Part model, mm, in its own coordinate system. A direction names the side the tool comes from. Give positions to 0.01 mm unless a question says otherwise; leave off trailing zeros. Loops run counter-clockwise (first coordinate to the right, second up) from the corner with the lowest first, then second, coordinate; pieces in that order, holes last. Notation, with made-up numbers: (58.25, 16) -> (85.25, 16) arc R24 cw to (85.25, 28) -> close; hole circle Ø11 at (-5.5, 2.25). An arc over 180 degrees is marked (long way). One line per question, with ' | ' between items.
```python
from build123d import *

# Parameters (mm, degrees)
SKETCH_1_W               = 45.9
SKETCH_1_H               = 49.9
EXTRUDE_1_DEPTH          = 6
SKETCH_2_R               = 1.9
EXTRUDE_2_DEPTH          = 8.9
EXTRUDE_START            = -8.9
SKETCH_3_R               = 1.9
EXTRUDE_3_DEPTH          = 8.9
FILLET_3_R               = 10
CUT_EXTRUDE_START        = -10
SKETCH_6_R               = 1.9
CUT_EXTRUDE_2_DEPTH      = 10
SKETCH_7_W               = 45.9
SKETCH_7_H               = 49.9
CUT_EXTRUDE_3_DEPTH      = 5
FILLET_4_R               = 4
SKETCH_8_W               = 28.1
SKETCH_8_H               = 49.9
EXTRUDE_5_DEPTH          = 5
FILLET_5_R               = 2
SKETCH_11_R              = 2.25
CUT_EXTRUDE_4_DEPTH      = 31
CUT_EXTRUDE_1_DEPTH      = 66
CUT_EXTRUDE_1_DEPTH_BACK = 70


with BuildPart() as part:
    # 草图1 → 凸台-拉伸1 (new body)
    with BuildSketch(Plane.XY):
        with Locations((22.95, -24.95)):
            Rectangle(SKETCH_1_W, SKETCH_1_H)
    extrude(amount=EXTRUDE_1_DEPTH)

    # 草图2 → 凸台-拉伸2 (add)
    with BuildSketch(Plane(origin=(45.9, 0, 0), x_dir=(0, 0, -1), z_dir=(1, 0, 0))):
        with BuildLine():
            Line((-6, 0), (-17.3, 0))
            ThreePointArc((-17.3, 0), (-20.410567122, 4.633542967), (-24.02783532, 8.883333436))
            ThreePointArc((-24.02783532, 8.883333436), (-33.92465453, 9.113485719), (-34.154806758, -0.783333492))
            ThreePointArc((-34.154806758, -0.783333492), (-24.472236128, -24.949999926), (-34.154806656, -49.116666401))
            ThreePointArc((-34.154806656, -49.116666401), (-33.924654493, -59.013485754), (-24.027835147, -58.783333255))
            ThreePointArc((-24.027835147, -58.783333255), (-20.410567046, -54.533542867), (-17.3, -49.9))
            Line((-17.3, -49.9), (-6, -49.9))
            Line((-6, -49.9), (-6, 0))
        make_face()
        with Locations(Location((-16.972236128, -24.95, 0), (0, 0, 90))):
            Circle(SKETCH_2_R, mode=Mode.SUBTRACT)
        with Locations(Location((-29.420197927, 5.1020382, 0), (0, 0, 90))):
            Circle(SKETCH_2_R, mode=Mode.SUBTRACT)
        with Locations(Location((-29.420197927, -55.0020382, 0), (0, 0, 90))):
            Circle(SKETCH_2_R, mode=Mode.SUBTRACT)
    extrude(amount=-EXTRUDE_2_DEPTH)

    # 草图3 → 凸台-拉伸3 (add)
    with BuildSketch(Plane.ZY.offset(EXTRUDE_START)):
        with BuildLine():
            Line((6, -49.9), (17.3, -49.9))
            ThreePointArc((17.3, -49.9), (62.08503163, -73.880290206), (104.061658089, -45.267072848))
            ThreePointArc((104.061658089, -45.267072848), (100.098824974, -34.670094153), (89.501846395, -38.63292758))
            ThreePointArc((89.501846395, -38.63292758), (26.472236128, -24.950000045), (89.501846358, -11.267072337))
            ThreePointArc((89.501846358, -11.267072337), (100.09882522, -15.229905735), (104.061657827, -4.632926576))
            ThreePointArc((104.061657827, -4.632926576), (62.085031314, 23.980290223), (17.3, 0))
            Line((17.3, 0), (6, 0))
            Line((6, 0), (6, -49.9))
        make_face()
        with Locations(Location((90.93848789, 6.516251763, 0), (0, 0, 270))):
            Circle(SKETCH_3_R, mode=Mode.SUBTRACT)
        with Locations(Location((28.005984365, -56.416251763, 0), (0, 0, 270))):
            Circle(SKETCH_3_R, mode=Mode.SUBTRACT)
        with Locations(Location((16.972236128, -24.95, 0), (0, 0, 90))):
            Circle(SKETCH_3_R, mode=Mode.SUBTRACT)
        with Locations(Location((59.472236128, -69.45, 0), (0, 0, 270))):
            Circle(SKETCH_3_R, mode=Mode.SUBTRACT)
        with Locations(Location((90.93848789, -56.416251763, 0), (0, 0, 270))):
            Circle(SKETCH_3_R, mode=Mode.SUBTRACT)
        with Locations(Location((28.005984365, 6.516251763, 0), (0, 0, 270))):
            Circle(SKETCH_3_R, mode=Mode.SUBTRACT)
        with Locations(Location((59.472236128, 19.55, 0), (0, 0, 270))):
            Circle(SKETCH_3_R, mode=Mode.SUBTRACT)
    extrude(amount=EXTRUDE_3_DEPTH)

    # 圆角3
    fillet_3_edges = [part.edges().sort_by_distance(p)[0] for p in [
        (41.45, 0, 17.3),
        (41.45, -49.9, 17.3),
        (4.45, -49.9, 17.3),
        (4.45, 0, 17.3),
    ]]
    fillet(fillet_3_edges, radius=FILLET_3_R)

    # 草图6 → 切除-拉伸2 (cut)
    # profile 1 of 2: a face of its own
    with BuildSketch(Plane.ZY.offset(CUT_EXTRUDE_START)):
        with BuildLine():
            ThreePointArc((104.061657942, -4.632926829), (85.981321722, 16.260051941), (59.472232168, 24.05))
            ThreePointArc((59.472232168, 24.05), (65.12908684, 21.706854481), (67.472232822, 16.05))
            ThreePointArc((67.472232822, 16.05), (65.129087169, 10.393145848), (59.472233099, 8.05))
            ThreePointArc((59.472233099, 8.05), (77.32529362, 2.803708548), (89.501846738, -11.267073171))
            ThreePointArc((89.501846738, -11.267073171), (100.098825511, -15.229905602), (104.061657942, -4.632926829))
        make_face()
        with Locations((90.93848789, 6.516251763)):
            Circle(SKETCH_6_R, mode=Mode.SUBTRACT)
    # profile 2 of 2: a face of its own
    with BuildSketch(Plane.ZY.offset(CUT_EXTRUDE_START)):
        with BuildLine():
            ThreePointArc((89.501846738, -38.632926829), (77.325293679, -52.70370851), (59.472233238, -57.95))
            ThreePointArc((59.472233238, -57.95), (65.129087219, -60.293145898), (67.472232822, -65.95))
            ThreePointArc((67.472232822, -65.95), (65.129086835, -71.606854486), (59.472232153, -73.95))
            ThreePointArc((59.472232153, -73.95), (85.981321716, -66.160051945), (104.061657942, -45.267073171))
            ThreePointArc((104.061657942, -45.267073171), (100.098825511, -34.670094398), (89.501846738, -38.632926829))
        make_face()
        with Locations((90.93848789, -56.416251763)):
            Circle(SKETCH_6_R, mode=Mode.SUBTRACT)
    extrude(amount=CUT_EXTRUDE_2_DEPTH, mode=Mode.SUBTRACT)


with BuildPart() as cut_extrude_2_kept_piece:
    # of the separate pieces the step leaves, the one the design keeps (cut_extrude_2_pieces_kept)
    add(part.part.solids().sort_by_distance((0, 0, 11.938064209))[0])

    # 草图7 → 切除-拉伸3 (cut)
    with BuildSketch(Plane(origin=(0, 0, 0), x_dir=(-1, 0, 0), z_dir=(0, 0, -1))):
        with Locations((-22.95, -24.95)):
            Rectangle(SKETCH_7_W, SKETCH_7_H)
    extrude(amount=-CUT_EXTRUDE_3_DEPTH, mode=Mode.SUBTRACT)

    # 圆角4
    fillet_4_edges = [cut_extrude_2_kept_piece.edges().sort_by_distance(p)[0] for p in [
        (45.9, -24.95, 5),
        (0, -24.95, 5),
    ]]
    fillet(fillet_4_edges, radius=FILLET_4_R)

    # 草图8 → 凸台-拉伸5 (add)
    with BuildSketch(Plane.XY.offset(6)):
        with Locations((22.95, -24.95)):
            Rectangle(SKETCH_8_W, SKETCH_8_H)
    extrude(amount=EXTRUDE_5_DEPTH)

    # 圆角5
    fillet_5_edges = [cut_extrude_2_kept_piece.edges().sort_by_distance(p)[0] for p in [
        (37, -24.95, 11),
        (8.9, -24.95, 11),
    ]]
    fillet(fillet_5_edges, radius=FILLET_5_R)

    # 草图11 → 切除-拉伸4 (cut)
    with BuildSketch(Plane.XY.offset(11)):
        with Locations((22.95, -7.7)):
            Circle(SKETCH_11_R)
        with Locations((22.95, -42.2)):
            Circle(SKETCH_11_R)
    extrude(amount=-CUT_EXTRUDE_4_DEPTH, mode=Mode.SUBTRACT)

    # 草图4 → 切除-拉伸1 (cut, two sides: drawn at the far end of the back side and taken through both)
    with BuildSketch(Plane.XY.offset(6).offset(-CUT_EXTRUDE_1_DEPTH_BACK)):
        with BuildLine():
            ThreePointArc((28.95, -24.95), (27.192640687, -20.707359313), (22.95, -18.95))
            Line((22.95, -18.95), (22.95, -30.95))
            ThreePointArc((22.95, -30.95), (27.192640687, -29.192640687), (28.95, -24.95))
        make_face()
        with BuildLine():
            Line((22.95, -30.95), (22.95, -18.95))
            ThreePointArc((22.95, -18.95), (16.95, -24.95), (22.95, -30.95))
        make_face()
    extrude(amount=CUT_EXTRUDE_1_DEPTH + CUT_EXTRUDE_1_DEPTH_BACK, mode=Mode.SUBTRACT)

    # 草图12 → 切除-旋转1 (revolve, cut)
    with BuildSketch(Plane.ZY.offset(-22.95), mode=Mode.PRIVATE) as cut_revolve_1_sk:
        Polygon((8.4, -7.7), (11, -7.7), (11, -5.45), (11, -3.7), (8.4, -5.6), align=None)
    cut_revolve_1 = revolve(cut_revolve_1_sk.sketch.rotate(Axis((22.95, -7.7, 5), (0, 0, 1)), 270), axis=Axis((22.95, -7.7, 5), (0, 0, 1)), mode=Mode.SUBTRACT)

    # 镜向2: 切除-旋转1 across plane
    add(cut_revolve_1.mirror(Plane.ZX.offset(-24.95)), mode=Mode.SUBTRACT)


solid = cut_extrude_2_kept_piece.part
```
1) Saw through at A-A (y = -20). Give the cut face in (x, z).
Found:
outline: (0, 9) arc R4 ccw to (4, 5) -> (19.56, 5) -> (19.56, 11) -> (10.9, 11) arc R2 cw to (8.9, 13) -> (8.9, 26.85) -> (0, 26.85) -> close; (26.34, 5) -> (41.9, 5) arc R4 ccw to (45.9, 9) -> (45.9, 24.82) -> (37, 24.82) -> (37, 13) arc R2 cw to (35, 11) -> (26.34, 11) -> close
2) Saw through at B-B (z = 49). Give the cut face in (x, y).
Found:
outline: (0, -72.82) -> (8.9, -72.82) -> (8.9, -56.24) -> (0, -56.24) -> close; (0, 6.34) -> (8.9, 6.34) -> (8.9, 22.92) -> (0, 22.92) -> close
3) Saw through at D-D (y = -7.7). Give the cut face in (x, z).
Found:
outline: (0, 9) arc R4 ccw to (4, 5) -> (20.7, 5) -> (20.7, 8.61) -> (18.95, 11) -> (10.9, 11) arc R2 cw to (8.9, 13) -> (8.9, 31.34) -> (0, 31.34) -> close; (25.2, 5) -> (41.9, 5) arc R4 ccw to (45.9, 9) -> (45.9, 29.02) -> (37, 29.02) -> (37, 13) arc R2 cw to (35, 11) -> (26.95, 11) -> (25.2, 8.61) -> close
4) Tool access for faces 1 (the cylindrical face through (4.512, 18.916, 37.638)), 2 (the cylindrical face through (4.51, -54.91, 26.85)), 3 (the flat face through (8.9, -13, 28)): list every direction of +Z, -Z, +X, -X, +Y, -Y with a clear straight run to the whole face (end or side of a thin tool).
Found:
face 1: -Z, +X, -X, +Y | face 2: -X | face 3: +Z, +Y, -Y
5) Drill centre lines: line 1 (Y direction, x = 22.95, z = 7.6); line 2 (X direction, y = -15.5, z = 24); line 3 (Z direction, x = 6, y = -24.95). Where is each one in solid material? Low to high.
Found:
line 1: -49.9 to -44.45, -39.95 to -30.95, -18.95 to -9.95, -5.45 to 0 | line 2: 0 to 8.9, 37 to 45.9 | line 3: 5 to 15.07, 18.87 to 26.47
6) Pin check, flat tips, straight feed: P1, Ø7.5, axis at x = 23, z = 7.5, coming from the +Y side; P2, Ø1, axis at x = 39.5, y = 6, coming from the +Z side; P3, Ø5, axis at y = 5.1, z = 29.42, coming from the -X side; P4, Ø12, axis at x = 20.5, y = -28, coming from the +Z side. Stop position of each tip, or through.
Found:
P1: y = 0 | P2: z = 35.94 | P3: x = 0 | P4: z = 11
7) Saw through at C-C (y = -69.45). Give the cut face in (x, z).
Found:
outline: (0, 38.96) -> (8.9, 38.96) -> (8.9, 57.57) -> (0, 57.57) -> close; (0, 61.37) -> (8.9, 61.37) -> (8.9, 66.67) -> (0, 66.67) -> close
8) Pull direction X, two halves, no side cores. Call faces 4 (the cylindrical face through (41.51, -53.25, 28.69)), 5 (the cylindrical face through (22.462, -44.396, 6.828)), 6 (the flat face through (45.9, -24, 20)), 7 (the cylindrical face through (9.5, -24.6, 11.57)): pulls with the +X half, pulls with the -X half, needs draft (parallel to the pull), parting line crosses it, or undercut.
Found:
face 4: needs draft | face 5: undercut | face 6: pulls with the +X half | face 7: undercut
